Design review of the part built by this model. Coordinates are the model's own, in mm. Face numbers are marked on the shaded views. A direction names the side the tool comes from. Round coordinates to 2 decimals unless told otherwise and drop trailing zeros. Order: outer loops, then holes, each group sorted by start corner. A loop starts at its lowest first (then second) coordinate and runs counter-clockwise, first axis right, second up. Notation, with made-up numbers: M -3,-27 L 56,-27 A36 ccw 56,7 Z; hole C 39.25,16 d11. An arc over 180 degrees is marked long. Write item = value, one per line. Start each with the question number.
```python
from build123d import *

# Parameters (mm, degrees)
SKETCH_1_W          = 5
SKETCH_1_H          = 4
SKETCH_2_R          = 28.5
EXTRUDE_1_DEPTH     = 2.5
SKETCH_3_R          = 2
CUT_EXTRUDE_1_DEPTH = 2


with BuildPart() as part:
    # 草图1 → 旋转1 (revolve)
    with BuildSketch(Plane.XY, mode=Mode.PRIVATE) as revolve_1_sk:
        with Locations((2.5, 22.5)):
            Rectangle(SKETCH_1_W, SKETCH_1_H)
        Polygon((0, 20.5), (0, 14), (8.5, 14), (8.5, 20.5), (5, 20.5), align=None)
        Polygon((0, 14), (0, 12.5), (10, 12.5), (10, 14), (8.5, 14), align=None)
        with BuildLine():
            Line((0, 12.5), (0, 11.6))
            Line((0, 11.6), (18, 11.6))
            add(Edge.make_bspline(
                [(18, 11.6), (16.79764846, 12.364408857), (15.52083483, 12.5), (14.156281908, 12.5)],
                knots=[0, 0, 0, 0, 1, 1, 1, 1], degree=3))
            Line((14.156281908, 12.5), (10, 12.5))
            Line((10, 12.5), (0, 12.5))
        make_face()
        Polygon((0, 11.6), (0, 2.006476073), (27.5, 2.006476073), (18, 11.6), align=None)
        with BuildLine():
            Line((0, 2.006476073), (0, 0))
            Line((0, 0), (28.5, 0))
            add(Edge.make_bspline(
                [(28.5, 0), (28.41881975, 1.211999363), (27.5, 2.006476073)],
                knots=[0, 0, 0, 1, 1, 1], degree=2))
            Line((27.5, 2.006476073), (0, 2.006476073))
        make_face()
    revolve(revolve_1_sk.sketch.rotate(Axis((0, 0, 0), (0, 1, 0)), 90), axis=Axis((0, 0, 0), (0, 1, 0)))

    # 草图2 → 凸台-拉伸1 (add)
    with BuildSketch(Plane.XZ):
        with Locations(Location((0, 0, 0), (0, 0, 270))):
            Circle(SKETCH_2_R)
    extrude(amount=EXTRUDE_1_DEPTH)

    # 草图3 → 切除-拉伸1 (cut)
    with BuildSketch(Plane(origin=(0, 24.5, 0), x_dir=(1, 0, 0), z_dir=(0, 1, 0))):
        with Locations(Location((0, 0, 0), (0, 0, 270))):
            Circle(SKETCH_3_R)
    extrude(amount=-CUT_EXTRUDE_1_DEPTH, mode=Mode.SUBTRACT)


solid = part.part
```
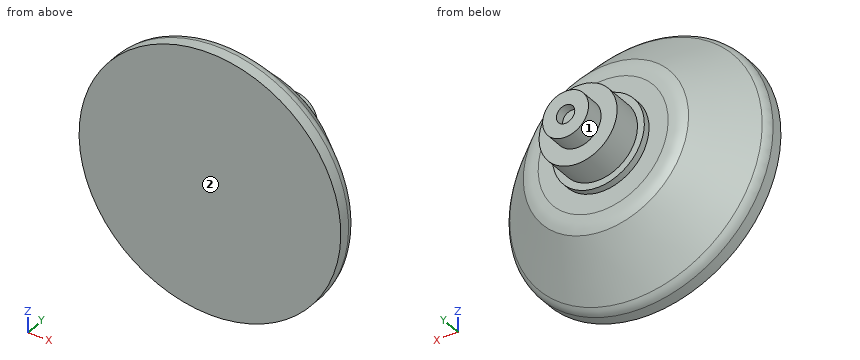
(1) For the marked faces 1 and 2, list the 3-axis set-ups (+Z, -Z, +X, -X, +Y, -Y) from which the entire face can be reached by the end or side of a thin tool; tool diameter is ignored.
(2) Consider section A-A, the plane y = 10. Write out the cut boundary in (x, z).
(3) For line 1 along X through (y, z) = (22.9, 0); line 2 along Z through (x, y) = (-1.5, 23.25); line 3 along X through (y, z) = (1.5, 24.5), list the stretches that pass through material, from the lowest coordinate up. Write a range as [from, to].
(4) Insertion check: pin 1 (10 mm diameter, centred on y = 14, z = -8.5, fed in from +X); pin 2 (5 mm diameter, centred on y = 10, z = -2, fed in from +X); pin 3 (2 mm diameter, centred on y = 19, z = -5.5, fed in from +X). Each pin has a flat end and moves straight along its axis. Give the tip position at first contact, or say it passes through.
(5) Consider section B-B, the plane y = 6.75. Write out the cut boundary in (x, z).
Completed:
q1.face_1 = +Y
q1.face_2 = +Z, -Z, +X, -X, -Y
q2.outline = C 0,0 d39.17
q3.line_1 = [-5, -2], [2, 5]
q3.line_2 = [-4.77, -1.32], [1.32, 4.77]
q3.line_3 = [-13.49, 13.49]
q4.pin_1 = 19.11
q4.pin_2 = 21.98
q4.pin_3 = 7.21
q5.outline = C 0,0 d45.61
